```python
from build123d import *

# Parameters (mm, degrees)
SKETCH1_R            = 6.35
SKETCH1_R_2          = 3.2639
SKETCH1_R_3          = 2.1463
BOSS_EXTRUDE1_DEPTH  = 6.35
FILLET1_R            = 6.35
FILLET2_R            = 6.35
FILLET1_OF_MIRROR1_R = 6.35
FILLET2_OF_MIRROR1_R = 6.35


with BuildPart() as part:
    # Sketch1 → Boss-Extrude1 (new body)
    # profile 1 of 5: a face of its own
    with BuildSketch(Plane(origin=(0, 0, -190.5), x_dir=(-1, 0, 0), z_dir=(0, 0, -1))):
        with BuildLine():
            Line((-222.25, 270.076638938), (-222.25, 187.123361062))
            ThreePointArc((-222.25, 187.123361062), (-216.773935033, 185.995115786), (-214.3125, 180.975))
            ThreePointArc((-214.3125, 180.975), (-216.773935033, 175.954884214), (-222.25, 174.826638938))
            Line((-222.25, 174.826638938), (-222.25, 127))
            Line((-222.25, 127), (0, 127))
            Line((0, 127), (0, 139.7))
            Line((0, 139.7), (-150.8125, 139.7))
            ThreePointArc((-150.8125, 139.7), (-158.964771181, 140.358395772), (-166.90572658, 142.316516748))
            ThreePointArc((-166.90572658, 142.316516748), (-171.738540659, 141.672571795), (-174.60521092, 145.616295752))
            ThreePointArc((-174.60521092, 145.616295752), (-194.340133262, 164.308681923), (-201.6125, 190.5))
            Line((-201.6125, 190.5), (-201.6125, 282.575))
            Line((-201.6125, 282.575), (-220.6625, 282.575))
            ThreePointArc((-220.6625, 282.575), (-216.172371939, 280.715128061), (-214.3125, 276.225))
            ThreePointArc((-214.3125, 276.225), (-216.773935033, 271.204884214), (-222.25, 270.076638938))
        make_face()
    # profile 2 of 5: a face of its own
    with BuildSketch(Plane(origin=(0, 0, -190.5), x_dir=(-1, 0, 0), z_dir=(0, 0, -1))):
        with Locations((-220.6625, 276.225)):
            Circle(SKETCH1_R)
        with Locations((-220.6625, 276.225)):
            Circle(SKETCH1_R_2, mode=Mode.SUBTRACT)
    # profile 3 of 5: a face of its own
    with BuildSketch(Plane(origin=(0, 0, -190.5), x_dir=(-1, 0, 0), z_dir=(0, 0, -1))):
        with Locations((-220.6625, 180.975)):
            Circle(SKETCH1_R)
        with Locations((-220.6625, 180.975)):
            Circle(SKETCH1_R_2, mode=Mode.SUBTRACT)
    # profile 4 of 5: a face of its own
    with BuildSketch(Plane(origin=(0, 0, -190.5), x_dir=(-1, 0, 0), z_dir=(0, 0, -1))):
        with BuildLine():
            ThreePointArc((-165.1, 146.05), (-170.079577741, 150.807550158), (-174.60521092, 145.616295752))
            ThreePointArc((-174.60521092, 145.616295752), (-170.823600368, 143.807432475), (-166.90572658, 142.316516748))
            ThreePointArc((-166.90572658, 142.316516748), (-165.575132529, 143.976383252), (-165.1, 146.05))
        make_face()
        with Locations((-169.8625, 146.05)):
            Circle(SKETCH1_R_3, mode=Mode.SUBTRACT)
    # profile 5 of 5: a face of its own
    with BuildSketch(Plane(origin=(0, 0, -190.5), x_dir=(-1, 0, 0), z_dir=(0, 0, -1))):
        with BuildLine():
            ThreePointArc((-166.90572658, 142.316516748), (-170.823600368, 143.807432475), (-174.60521092, 145.616295752))
            ThreePointArc((-174.60521092, 145.616295752), (-171.738540659, 141.672571795), (-166.90572658, 142.316516748))
        make_face()
    boss_extrude1 = extrude(amount=BOSS_EXTRUDE1_DEPTH)

    # Fillet1
    fillet1_edges = [part.edges().sort_by_distance(p)[0] for p in [
        (174.60521092, 145.616295752, -193.675),
        (166.90572658, 142.316516748, -193.675),
    ]]
    fillet(fillet1_edges, radius=FILLET1_R)

    # Fillet2
    fillet2_edges = [part.edges().sort_by_distance(p)[0] for p in [
        (222.25, 174.826638938, -193.675),
        (222.25, 187.123361062, -193.675),
        (222.25, 270.076638938, -193.675),
        (201.6125, 282.575, -193.675),
    ]]
    fillet(fillet2_edges, radius=FILLET2_R)

    # Mirror1: Boss-Extrude1 across plane
    add(boss_extrude1.mirror(Plane(origin=(0, 0, 0), x_dir=(0, 0, 1), z_dir=(1, 0, 0))))

    # Fillet1 of Mirror1
    fillet1_of_mirror1_edges = [part.edges().sort_by_distance(p)[0] for p in [
        (-174.60521092, 145.616295752, -193.675),
        (-166.90572658, 142.316516748, -193.675),
    ]]
    fillet(fillet1_of_mirror1_edges, radius=FILLET1_OF_MIRROR1_R)

    # Fillet2 of Mirror1
    fillet2_of_mirror1_edges = [part.edges().sort_by_distance(p)[0] for p in [
        (-222.25, 174.826638938, -193.675),
        (-222.25, 187.123361062, -193.675),
        (-222.25, 270.076638938, -193.675),
        (-201.6125, 282.575, -193.675),
    ]]
    fillet(fillet2_of_mirror1_edges, radius=FILLET2_OF_MIRROR1_R)


solid = part.part
```
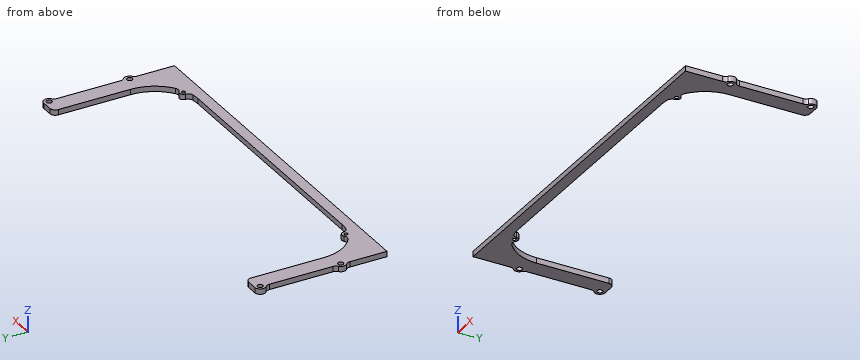
CAD build for the part. Positions are in the model's coordinates, mm. Round coordinates to 2 decimals unless told otherwise and drop trailing zeros. Write each loop counter-clockwise with the first axis right and the second up, starting at its lowest first coordinate (ties: lowest second). Pieces come first, ordered by that corner, then holes. Notation, with made-up numbers: M -24.75,77 L -19.75,77 A18 ccw -19.75,111 Z; hole C 89.5,-23 d3. An arc over 180 degrees is marked long. One line per question, with ' | ' between items.
1. Pin check, flat tips, straight feed: pin 1 Ø2 at (x, z) = (35.5, -193.5) entering from +Y; pin 2 Ø3 at (y, z) = (177, -193.5) entering from -X; pin 3 Ø1.9 at (y, z) = (224.5, -195) entering from +X; pin 4 Ø4 at (x, y) = (169.86, 146.05) entering from +Z. Stop position of each tip, or through.
Working result:
pin 1: y = 139.7 | pin 2: x = -226.51 | pin 3: x = 222.25 | pin 4: through
2. Cut at A-A on y = 237. Write the cut outline in (x, z), and give its area (3 significant figures).
Working result:
outline: M -222.25,-196.85 L -201.61,-196.85 L -201.61,-190.5 L -222.25,-190.5 Z; M 201.61,-196.85 L 222.25,-196.85 L 222.25,-190.5 L 201.61,-190.5 Z | area: 262 mm2
3. Probe L1, parallel to X at y = 247.5, z = -192.75; L2, parallel to Y at x = -27.5, z = -196.25; L3, parallel to X at y = 158.5, z = -195.5. List the from-to ranges inside material, lowest first. Write a range as from..to.
Working result:
L1: -222.25..-201.61, 201.61..222.25 | L2: 127..139.7 | L3: -222.25..-190.27, 190.27..222.25
4. Cut at C-C on z = -194.5. Count the separate pieces of the cut face and the enclosed holes in it, and give its area (3 significant figures).
Working result:
separate pieces: 1 | enclosed holes: 6 | area: 12,800 mm2
5. Cut at B-B on x = -10.5. Write the cut outline in (y, z).
Working result:
outline: M 127,-196.85 L 139.7,-196.85 L 139.7,-190.5 L 127,-190.5 Z
